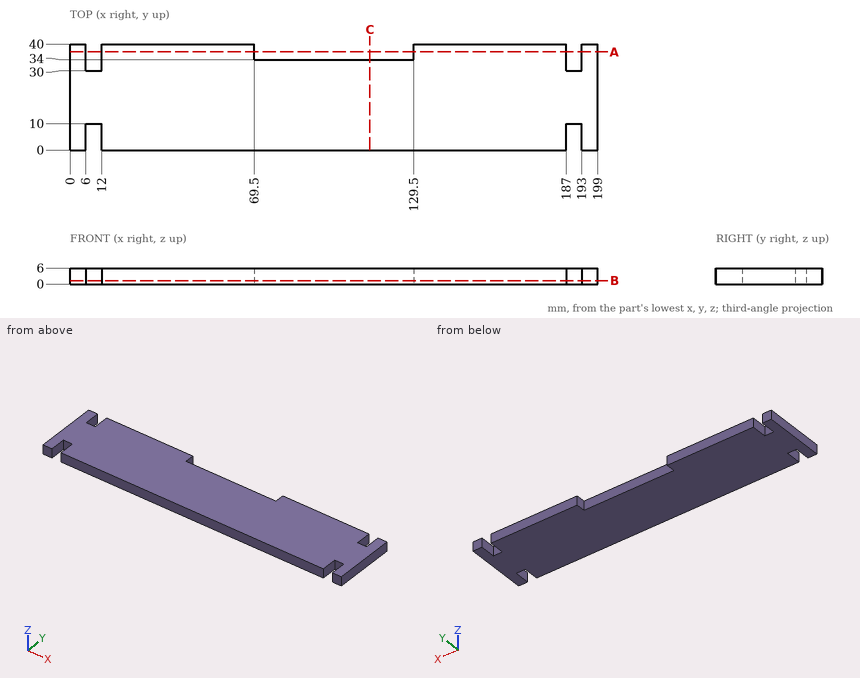
Verification items for this drawing (mm, ordinates from the low corner). Round coordinates to 2 decimals unless told otherwise and drop trailing zeros. Order: outer loops, then holes, each group sorted by start corner. A loop starts at its lowest first (then second) coordinate and runs counter-clockwise, first axis right, second up. Notation, with made-up numbers: (-11, 47.5) - (38, 47.5) arc R25 cw to (38, 69.5) - close; hole circle Ø4 at (1, 60.5). An arc over 180 degrees is marked (long way). Use CSV: the item, a comma, the result in double quotes. Start each with the question number.
1) Go/stop test with flat-tipped pins: P1, Ø1.8, axis at x = 10, z = 1.5, coming from the +Y side; P2, Ø1.8, axis at x = 90, z = 2.5, coming from the +Y side. Record where each tip stops, or that it passes through.
2) Thickness scan on L1, parallel to X at y = 4.5, z = 4.25; L2, parallel to X at y = 36, z = 2.85; L3, parallel to Y at x = 191.5, z = 2.2. Record the ranges inside material, lowest first.
3) Section check B-B, the plane z = 1.3. Record the cut outline in (x, y).
4) Section check A-A, the plane y = 37. Record the cut outline in (x, z).
5) Section check C-C, the plane x = 113. Record the cut outline in (y, z), plus the area to 3 significant figures.
Answers:
1,P1,"stops at y = 30"
1,P2,"stops at y = 34"
2,L1,"x = 0 to 6, 12 to 187, 193 to 199"
2,L2,"x = 0 to 6, 12 to 69.5, 129.5 to 187, 193 to 199"
2,L3,"y = 10 to 30"
3,outline,"(0, 0) - (6, 0) - (6, 10) - (12, 10) - (12, 0) - (187, 0) - (187, 10) - (193, 10) - (193, 0) - (199, 0) - (199, 40) - (193, 40) - (193, 30) - (187, 30) - (187, 40) - (129.5, 40) - (129.5, 34) - (69.5, 34) - (69.5, 40) - (12, 40) - (12, 30) - (6, 30) - (6, 40) - (0, 40) - close"
4,outline,"(0, 0) - (6, 0) - (6, 6) - (0, 6) - close; (12, 0) - (69.5, 0) - (69.5, 6) - (12, 6) - close; (129.5, 0) - (187, 0) - (187, 6) - (129.5, 6) - close; (193, 0) - (199, 0) - (199, 6) - (193, 6) - close"
5,outline,"(0, 0) - (34, 0) - (34, 6) - (0, 6) - close"
5,area,"204 mm²"
